from build123d import *

# Parameters (mm, degrees)
F1_DEPTH = 10
F2_R     = 3
F4_R     = 4.5
F5_DEPTH = 22.6211939253
F6_R     = 2.25
F7_DEPTH = 2.0010001


with BuildPart() as f1:
    # F0 (on Front) → F1 (new body, symmetric)
    with BuildSketch(Plane.XZ):
        with BuildLine():
            add(Edge.make_bspline(
                [(0, 12), (66.9550430253, -1.9531170396), (93.0146408351, -3.1716877372), (100, 24.6201938253)],
                knots=[0, 0, 0, 0, 84.8143811399, 84.8143811399, 84.8143811399, 84.8143811399], degree=3))
            Line((0, 12), (0, 0))
            Line((0, 0), (110, 0))
            Line((110, 0), (105.6587955583, 24.6201938253))
            Line((105.6587955583, 24.6201938253), (100, 24.6201938253))
        make_face()
    extrude(amount=F1_DEPTH, both=True)

    # F2
    f2_edges = [f1.edges().sort_by_distance(p)[0] for p in [
        (0, 5, 12),
        (0, -5, 12),
        (100, 5, 24.620194),
        (100, -5, 24.620194),
        (105.658796, 0, 24.620194),
    ]]
    fillet(f2_edges, radius=F2_R)

    # F4 (on offset) → F5 (cut, through all)
    with BuildSketch(Plane.XY.offset(2)):
        with Locations((8, 0)):
            Circle(F4_R)
        with Locations((91.0959199238, 0)):
            Circle(F4_R)
    extrude(amount=F5_DEPTH, mode=Mode.SUBTRACT)

    # F6 (on offset) → F7 (cut, through all)
    with BuildSketch(Plane.XY.offset(2)):
        with Locations((91.0959199238, 0)):
            Circle(F6_R)
        with Locations((8, 0)):
            Circle(F6_R)
    extrude(amount=-F7_DEPTH, mode=Mode.SUBTRACT)


solid = f1.part
For this review, take the finished solid that the model builds, in its own axes (mm). A direction names the side the tool comes from. Round coordinates to 2 decimals unless told otherwise and drop trailing zeros. Write item = value, one per line. Start each with the question number.
(1) The part is to be moulded in two halves that separate along Y. For faces 1 (the face through (10, -2, 2)), 2 (the face through (108.075, -0.14, 10.916)), 3 (the face through (59, -10, 1)), say which applies: +Y half, -Y half, draft (parallel to the pull), parting line (faces both ways), or undercut.
(2) We need section A-A (z = 4.75). Give the number of separate pieces and of enclosed holes in the cut face, then the cut area to 3 significant figures.
(3) For faces 4 (the face through (93.174, -0.862, 1.014)), 5 (the face through (3.504, 0.198, 6.571)), list the 3-axis set-ups (+Z, -Z, +X, -X, +Y, -Y) from which the entire face can be reached by the end or side of a thin tool; tool diameter is ignored.
(4) Clearance check with flat-ended pins moving along their axes: pin 1 Ø2.5 at (x, y) = (9.5, 0.5) entering from +Z; pin 2 Ø10 at (x, z) = (78.5, 13.5) entering from +Y; pin 3 Ø11.5 at (x, y) = (8, 0) entering from -Z; pin 4 Ø6 at (x, y) = (34, 5) entering from +Z. State where each tip first meets the part, or that it passes through.
(5) For line 1 along Y through (x, z) = (8, 1.2); line 2 along Y through (x, z) = (8, 6.75); line 3 along Z through (x, y) = (63.5, 6.5), list the stretches that pass through material, from the lowest coordinate up.
Results found:
q1.face_1 = undercut
q1.face_2 = draft
q1.face_3 = -Y half
q2.separate_pieces = 2
q2.enclosed_holes = 2
q2.area = 1,170 mm²
q3.face_4 = +Z, -Z
q3.face_5 = +Z
q4.pin_1 = 2
q4.pin_2 = through
q4.pin_3 = 0
q4.pin_4 = 6.02
q5.line_1 = -10 to -2.25, 2.25 to 10
q5.line_2 = -10 to -4.5, 4.5 to 10
q5.line_3 = 0 to 2.38
